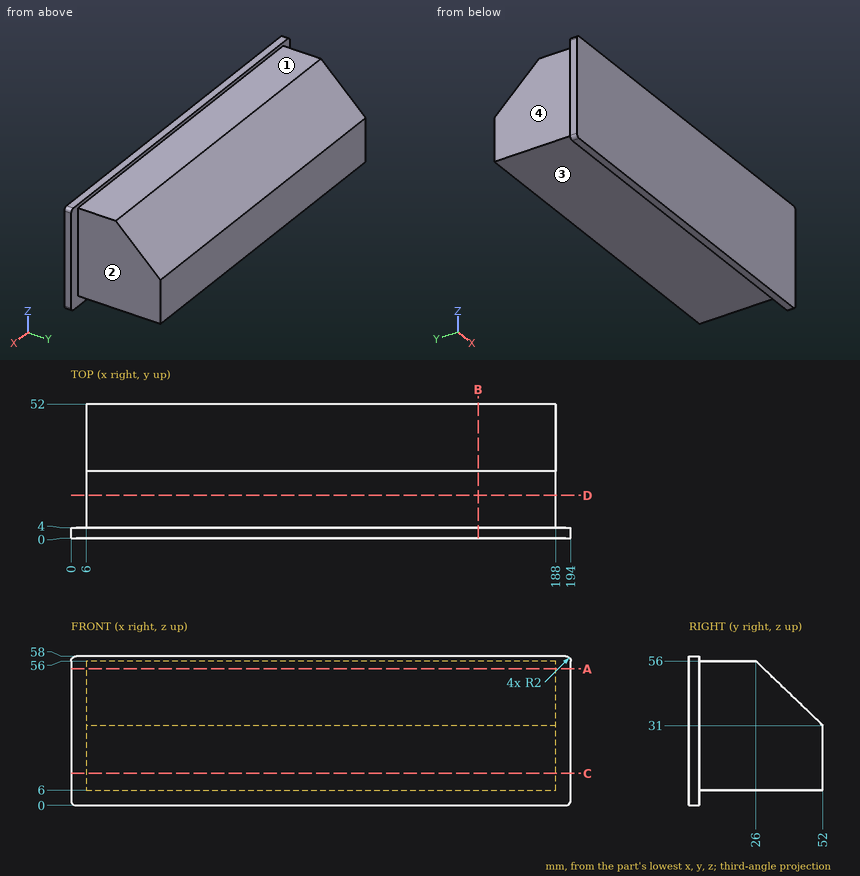
Answer from the drawing. Dimensions are ordinates in mm from the lowest x, y and z of the part. A direction names the side the tool comes from. Round coordinates to 2 decimals unless told otherwise and drop trailing zeros. Loops run counter-clockwise (first coordinate to the right, second up) from the corner with the lowest first, then second, coordinate; pieces in that order, holes last.
(1) The part is cut by section B-B, the plane x = 158. Give the vertices of the cut face in (y, z), and give its area (3 significant figures).
Computed values:
outline: (0, 0) - (4, 0) - (4, 6) - (52, 6) - (52, 31) - (26, 56) - (4, 56) - (4, 58) - (0, 58) - close
area: 2,310 mm2
(2) For the marked faces 1, 2, 3 and 4, determine the directions among +Z, -Z, +X, -X, +Y, -Y from which every point of the face is accessible in a straight line to the end or side of a thin tool.
Computed values:
face 1: +Z, +X, -X, +Y
face 2: +Z, -Z, +X, +Y
face 3: -Z, +X, -X, +Y
face 4: +Z, -Z, -X, +Y
(3) Each of these flat-tipped pins is pushed along its axis until it touches: P1, Ø12, axis at x = 117.5, z = 45.5, coming from the +Y side; P2, Ø24, axis at y = 24.5, z = 25, coming from the +X side; P3, Ø10, axis at x = 92.5, y = 23.5, coming from the -Z side. Where does it stop, or does it pass through?
Computed values:
P1: stops at y = 43.16
P2: stops at x = 188
P3: stops at z = 6
(4) Find the intervals of material crossed by L1, parallel to Z at x = 138, y = 10.5; L2, parallel to X at y = 40.5, z = 28; L3, parallel to Z at x = 148, y = 33, in increasing order.
Computed values:
L1: z = 6 to 56
L2: x = 6 to 188
L3: z = 6 to 49.27
(5) The part is cut by section C-C, the plane z = 12.5. Give the vertices of the cut face in (x, y).
Computed values:
outline: (0, 0) - (194, 0) - (194, 4) - (188, 4) - (188, 52) - (6, 52) - (6, 4) - (0, 4) - close
(6) The part is cut by section A-A, the plane z = 53. Give the vertices of the cut face in (x, y).
Computed values:
outline: (0, 0) - (194, 0) - (194, 4) - (188, 4) - (188, 29.12) - (6, 29.12) - (6, 4) - (0, 4) - close
(7) The part is cut by section D-D, the plane y = 16.5. Give the vertices of the cut face in (x, z).
Computed values:
outline: (6, 6) - (188, 6) - (188, 56) - (6, 56) - close
